from build123d import *

# Parameters (mm, degrees)
F5_DEPTH = 30
F6_DEPTH = 30


with BuildPart() as f5:
    # F1 (on offset) → F5 (new body)
    with BuildSketch(Plane.XY.offset(15)):
        Polygon((17.3205, 23.839623), (-17.3205, 23.839623), (-28.025158, -9.105926), (0, -29.467395), (28.025158, -9.105926), align=None)
    extrude(amount=-F5_DEPTH)

    # F3 (on offset) → F6 (join)
    with BuildSketch(Plane.XY.offset(-15)):
        Polygon((-17.3205, -23.839623), (17.3205, -23.839623), (28.025158, 9.105926), (0, 29.467395), (-28.025158, 9.105926), align=None)
    extrude(amount=F6_DEPTH)


solid = f5.part
Model file for the job. Use its own axes, mm. A direction names the side the tool comes from. Round coordinates to 2 decimals unless told otherwise and drop trailing zeros. Loops run counter-clockwise (first coordinate to the right, second up) from the corner with the lowest first, then second, coordinate; pieces in that order, holes last. Notation, with made-up numbers: M 84.25,-37 L 89.25,-37 A26 ccw 89.25,-4 Z; hole C 63.5,58.5 d6. An arc over 180 degrees is marked long. One line per question, with ' | ' between items.
1) Mould opens along Y. For faces 1 (the flat face through (24.21, 11.88, -0.21)), 2 (the flat face through (18.78, -19.35, -0.21)), 3 (the flat face through (0, 0, 15)), 4 (the flat face through (26.525, 4.489, -0.21)) say: +Y half, -Y half, draft (parallel to the pull), parting line (faces both ways), or undercut.
Solved:
face 1: +Y half | face 2: -Y half | face 3: draft | face 4: undercut
2) Band-saw the part on A-A (z = 11). Give the cut face in (x, y), then the cut area to 3 significant figures.
Solved:
outline: M -28.03,-9.11 L -20.28,-14.73 L -17.32,-23.84 L -7.75,-23.84 L 0,-29.47 L 7.75,-23.84 L 17.32,-23.84 L 20.28,-14.73 L 28.03,-9.11 L 25.07,0 L 28.03,9.11 L 20.28,14.73 L 17.32,23.84 L 7.75,23.84 L 0,29.47 L -7.75,23.84 L -17.32,23.84 L -20.28,14.73 L -28.03,9.11 L -25.07,0 Z | area: 2,280 mm²
3) 3-axis set-ups, long thin cutter, end or side, ignore diameter. For faces 5 (the flat face through (-13, -23.84, 0)), 6 (the flat face through (13, 23.84, 0)), 7 (the flat face through (-26.567, 4.617, -0.21)): which of +Z, -Z, +X, -X, +Y, -Y reach the whole face in a straight line?
Solved:
face 5: +Z, -Z, -X, -Y | face 6: +Z, -Z, +X, +Y | face 7: +Z, -Z, -X
4) Drill centre lines: line 1 along Y through (x, z) = (12, -0.75); line 2 along Y through (x, z) = (21, -11.75); line 3 along X through (y, z) = (11.5, -4.25). Where is each one in solid material? Low to high.
Solved:
line 1: y = -23.84 to 23.84 | line 2: y = -14.21 to 14.21 | line 3: x = -24.73 to 24.73
5) Flat gauge pins, fed straight in: pin 1 (4 mm diameter, centred on x = -11.5, z = 2, fed in from +Y); pin 2 (5 mm diameter, centred on x = -11, z = 2, fed in from -Y); pin 3 (5 mm diameter, centred on x = -3.5, z = 4, fed in from +Y). Where does each tip first touch, or does it go through?
Solved:
pin 1: stops at y = 23.84 | pin 2: stops at y = -23.84 | pin 3: stops at y = 28.74
6) Band-saw the part on B-B (x = -15.5). Give the cut face in (y, z).
Solved:
outline: M -23.84,-15 L 23.84,-15 L 23.84,15 L -23.84,15 Z
7) Band-saw the part on C-C (y = -4). Give the cut face in (x, z).
Solved:
outline: M -26.37,-15 L 26.37,-15 L 26.37,15 L -26.37,15 Z
